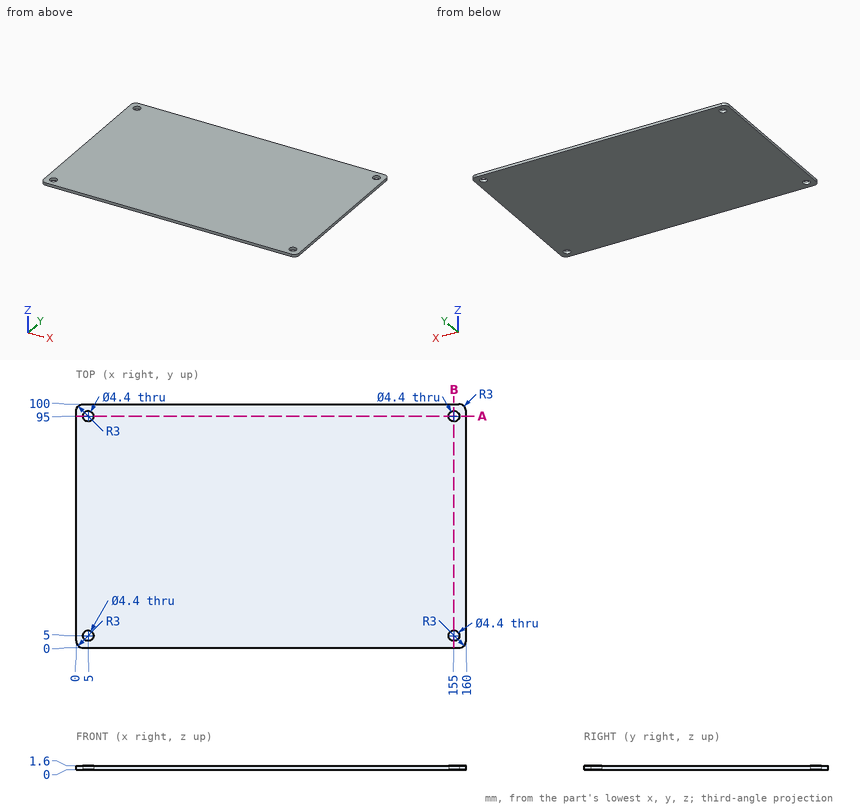
Input: dimensioned drawing with shaded views. Units: mm. Origin: part minimum x, y, z. Coordinates: 2 decimals unless noted, no trailing zeros. Loops run counter-clockwise (first coordinate to the right, second up) from the corner with the lowest first, then second, coordinate; pieces in that order, holes last.
Q1. Line query: line 1 along Y through (x, z) = (155, 0.5). Output: solid intervals per line, ascending.
Results are:
line 1: y = 0 to 2.8, 7.2 to 92.8, 97.2 to 100
Q2. Section A-A, the plane y = 95. Return the cut outline in (x, z).
Results are:
outline: (0, 0) - (2.8, 0) - (2.8, 1.6) - (0, 1.6) - close; (7.2, 0) - (152.8, 0) - (152.8, 1.6) - (7.2, 1.6) - close; (157.2, 0) - (160, 0) - (160, 1.6) - (157.2, 1.6) - close
Q3. Section B-B, the plane x = 155. Return the cut outline in (y, z).
Results are:
outline: (0, 0) - (2.8, 0) - (2.8, 1.6) - (0, 1.6) - close; (7.2, 0) - (92.8, 0) - (92.8, 1.6) - (7.2, 1.6) - close; (97.2, 0) - (100, 0) - (100, 1.6) - (97.2, 1.6) - close
Q4. Contact query for flat-ended pins moving along their axis: pin 1 (4 mm diameter, centred on x = 5, y = 95, fed in from -Z); pin 2 (1 mm diameter, centred on x = 99, y = 60.5, fed in from -Z). Output: stop coordinate, or through.
Results are:
pin 1: passes through
pin 2: stops at z = 0
